from build123d import *

# Parameters (mm, degrees)
F0_W      = 946.15
F0_H      = 533.4
F1_DEPTH  = 25.4
F2_W      = 215.9
F2_H      = 139.7
F3_DEPTH  = 25.4
F4_R      = 25.4
F5_W      = 946.15
F5_H      = 101.6
F6_DEPTH  = 25.4
F7_R      = 17.526
F8_DEPTH  = 50.801
F9_W      = 203.2
F9_H      = 127
F10_DEPTH = 6.35
F12_D     = 14.2875
F13_W     = 25.4
F13_H     = 501.65
F13_H_2   = 641.096
F14_DEPTH = 393.7
F16_DEPTH = 908.051
F18_DEPTH = 908.051


with BuildPart() as f1:
    # F0 (on Top) → F1 (new body)
    with BuildSketch(Plane.XY):
        Rectangle(F0_W, F0_H)
    extrude(amount=-F1_DEPTH)

    # F2 (on face) → F3 (join)
    with BuildSketch(Plane.XY):
        with Locations((-34.925, -336.55)):
            Rectangle(F2_W, F2_H)
    extrude(amount=-F3_DEPTH)

    # F4
    f4_edges = [f1.edges().sort_by_distance(p)[0] for p in [
        (-142.875, -266.7, -12.7),
        (73.025, -266.7, -12.7),
    ]]
    fillet(f4_edges, radius=F4_R)

    # F5 (on face) → F6 (join)
    with BuildSketch(Plane.XY):
        with Locations((0, 203.2)):
            Rectangle(F5_W, F5_H)
        with Locations((0, -203.2)):
            Rectangle(F5_W, F5_H)
    extrude(amount=F6_DEPTH)

    # F7 (on face) → F8 (cut, through all)
    with BuildSketch(Plane.XY.offset(25.4)):
        with Locations((-333.375, 203.2)):
            Circle(F7_R)
        with Locations((-333.375, -203.2)):
            Circle(F7_R)
        with Locations((263.525, -203.2)):
            Circle(F7_R)
        with Locations((263.525, 203.2)):
            Circle(F7_R)
    extrude(amount=-F8_DEPTH, mode=Mode.SUBTRACT)

    # F9 (on face) → F10 (join)
    with BuildSketch(Plane.XY):
        with Locations((-34.925, -336.55)):
            Rectangle(F9_W, F9_H)
    extrude(amount=F10_DEPTH)

    # F12 (through all)
    with Locations(Plane.XY.offset(6.35)):
        with Locations((-117.475, -292.1), (-117.475, -381), (47.625, -292.1), (47.625, -381)):
            Hole(F12_D / 2)

    # F13 (on face) → F14 (join)
    with BuildSketch(Plane(origin=(0, 0, -25.4), x_dir=(1, 0, 0), z_dir=(0, 0, -1))):
        with Locations((422.275, 3.175)):
            Rectangle(F13_W, F13_H)
        with Locations((-34.925, 72.898)):
            Rectangle(F13_W, F13_H_2)
        with Locations((-434.975, 3.175)):
            Rectangle(F13_W, F13_H)
    extrude(amount=F14_DEPTH)

    # F15 (on face) → F16 (cut, through all)
    with BuildSketch(Plane.YZ.offset(434.975)):
        Polygon((158.75, -419.1), (-393.446, -50.8), (-393.446, -419.1), align=None)
    extrude(amount=-F16_DEPTH, mode=Mode.SUBTRACT)

    # F17 (on face) → F18 (cut, through all)
    with BuildSketch(Plane.YZ.offset(434.975)):
        Polygon((155.575, -133.35), (155.575, -161.925), (222.25, -161.925), (247.65, -187.325), (247.65, -25.4), (206.375, -25.4), (206.375, -50.8), align=None)
    extrude(amount=-F18_DEPTH, mode=Mode.SUBTRACT)


solid = f1.part
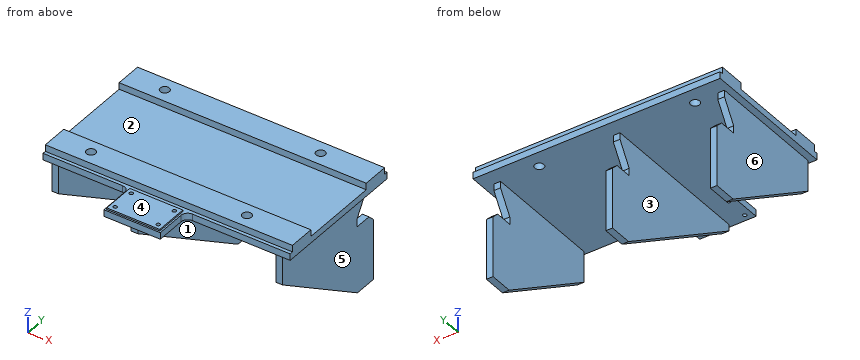
Read the model definition and answer for the solid it produces. Units are mm, in the model's axes. Face numbers are marked on the shaded views. A direction names the side the tool comes from. Coordinates: 2 decimals unless noted, no trailing zeros. Order: outer loops, then holes, each group sorted by start corner. A loop starts at its lowest first (then second) coordinate and runs counter-clockwise, first axis right, second up. Notation, with made-up numbers: (48, 54.25) -> (106, 54.25) arc R16 ccw to (106, 73.25) -> close; hole circle Ø2 at (69.25, -32.5). An arc over 180 degrees is marked (long way). Answer as a JSON object with one key per item and string values.
1) A cutting plane is placed at C-C, the plane x = -390. Determine the outline of the cut face in (y, z), plus the area to 3 significant figures.
Model answer:
{"outline": "(-266.7, -25.4) -> (266.7, -25.4) -> (266.7, 0) -> (254, 0) -> (254, 25.4) -> (152.4, 25.4) -> (152.4, 0) -> (-152.4, 0) -> (-152.4, 25.4) -> (-254, 25.4) -> (-254, 0) -> (-266.7, 0) -> close", "area": "18,700 mm²"}
2) A cutting plane is placed at D-D, the plane z = -313.5. Determine the outline of the cut face in (x, y) (3 decimals), plus the area to 3 significant figures.
Model answer:
{"outline": "(-447.675, 0.423) -> (-422.275, 0.423) -> (-422.275, 247.65) -> (-447.675, 247.65) -> close; (-47.625, 0.423) -> (-22.225, 0.423) -> (-22.225, 247.65) -> (-47.625, 247.65) -> close; (409.575, 0.423) -> (434.975, 0.423) -> (434.975, 247.65) -> (409.575, 247.65) -> close", "area": "18,800 mm²"}
3) The mould has two halves that part along Y. Classify the marked faces 1 and 2: released by +Y, released by -Y, zero draft, split by the parting line, or undercut.
Model answer:
{"face 1": "zero draft", "face 2": "undercut"}
4) A cutting plane is placed at A-A, the plane z = -210. Determine the outline of the cut face in (x, y) (3 decimals), plus the area to 3 significant figures.
Model answer:
{"outline": "(-447.675, -154.756) -> (-422.275, -154.756) -> (-422.275, 247.65) -> (-447.675, 247.65) -> close; (-47.625, -154.756) -> (-22.225, -154.756) -> (-22.225, 247.65) -> (-47.625, 247.65) -> close; (409.575, -154.756) -> (434.975, -154.756) -> (434.975, 247.65) -> (409.575, 247.65) -> close", "area": "30,700 mm²"}
5) A tool of negligible diameter and unlimited length cuts with its end or side. For the marked faces 3, 4, 5 and 6, from which of +Z, -Z, +X, -X, +Y, -Y can it reach the whole face along a straight path? Write none if from no direction.
Model answer:
{"face 3": "-Z, +Y, -Y", "face 4": "+Z, +X, -X, -Y", "face 5": "-Z, +X, +Y, -Y", "face 6": "-Z, -X, +Y, -Y"}
6) A cutting plane is placed at B-B, the plane y = -203.2. Determine the outline of the cut face in (x, z) (3 decimals), plus the area to 3 significant figures.
Model answer:
{"outline": "(-473.075, -25.4) -> (-447.675, -25.4) -> (-447.675, -177.689) -> (-422.275, -177.689) -> (-422.275, -25.4) -> (-350.901, -25.4) -> (-350.901, 25.4) -> (-473.075, 25.4) -> close; (-315.849, -25.4) -> (-47.625, -25.4) -> (-47.625, -177.689) -> (-22.225, -177.689) -> (-22.225, -25.4) -> (245.999, -25.4) -> (245.999, 25.4) -> (-315.849, 25.4) -> close; (281.051, -25.4) -> (409.575, -25.4) -> (409.575, -177.689) -> (434.975, -177.689) -> (434.975, -25.4) -> (473.075, -25.4) -> (473.075, 25.4) -> (281.051, 25.4) -> close", "area": "56,100 mm²"}
7) Each of these flat-tipped pins is pushed along its axis until it touches: pin 1 (2 mm diameter, centred on x = -135.5, y = 103, fed in from +Z); pin 2 (18.5 mm diameter, centred on x = -117.475, y = -381, fed in from -Z); pin 3 (12.5 mm diameter, centred on x = -431, z = -33, fed in from +Y) (3 decimals). Where does it stop, or does it pass through?
Model answer:
{"pin 1": "stops at z = 0", "pin 2": "stops at z = -25.4", "pin 3": "stops at y = 206.375"}
8) Consider line 1 along X through (y, z) = (42.5, -125.5) (3 decimals); line 2 along X through (y, z) = (-203, -2) (3 decimals); line 3 along Z through (x, y) = (-60, -118). Determine where each line is inside the solid, lowest interval first. Write a range as from..to.
Model answer:
{"line 1": "x = -447.675..-422.275, -47.625..-22.225, 409.575..434.975", "line 2": "x = -473.075..-350.9, -315.85..246, 281.05..473.075", "line 3": "z = -25.4..0"}
